Geometry: final body of the model. Coordinates: model frame, mm. A direction names the side the tool comes from. Give positions to 0.01 mm unless a question says otherwise; leave off trailing zeros. Write each loop counter-clockwise with the first axis right and the second up, starting at its lowest first coordinate (ties: lowest second). Pieces come first, ordered by that corner, then holes. Notation, with made-up numbers: M 54,14.25 L 109,14.25 A16 ccw 109,40.25 Z; hole C 33.25,18 d7. An arc over 180 degrees is marked long. Use a Markdown table: item, result. Add a question column.
(1) Reachability of faces 1 (the flat face through (2.2, 0, 0.1)), 2 (the cylindrical face through (0, 7, 5)), 3 (the cylindrical face through (-1.9, 4.3, -5.9)) from +Z, -Z, +X, -X, +Y, -Y: full face, straight path, thin tool, end or side. Return the list, or none.
(2) Material intervals for L1, parallel to X at y = 5.7, z = 0; L2, parallel to Z at x = -14, y = 24.5; L3, parallel to X at y = 19, z = -2.5, sorted ascending.
(3) Pin query (flat end, axial travel): pin 1 Ø16 at (x, z) = (0, 0) entering from +Y; pin 2 Ø12 at (x, y) = (-10.5, 13) entering from -Z; pin 3 Ø10 at (x, y) = (18, 26.5) entering from -Z. Return the tip coordinate at first contact, or that it passes through.
(4) Cut plane A-A (y = 19.25). Output: boundary loops of the cut face in (x, z).
(5) Cut plane B-B (y = 25). Output: boundary loops of the cut face in (x, z).
```python
from build123d import *

# Parameters (mm, degrees)
FILLET1_R = 5
FILLET2_R = 0.4
FILLET3_R = 1


with BuildPart() as part:
    # Sketch1 → Revolve1 (revolve)
    with BuildSketch(Plane.XY, mode=Mode.PRIVATE) as revolve1_sk:
        Polygon((5, 5.196152423), (5, 10), (25, 30), (26.697056275, 30), (6.2, 9.502943725), (6.2, 4.874613392), (6.2, 0), (2, 0), align=None)
    revolve(revolve1_sk.sketch.rotate(Axis((0, 0, 0), (0, 1, 0)), 90), axis=Axis((0, 0, 0), (0, 1, 0)))

    # Fillet1
    fillet1_edges = [part.edges().sort_by_distance(p)[0] for p in [
        (0, 9.502943725, 6.2),
        (0, 10, 5),
    ]]
    fillet(fillet1_edges, radius=FILLET1_R)

    # Fillet2
    fillet2_edges = [part.edges().sort_by_distance(p)[0] for p in [
        (0, 30, 26.697056275),
        (0, 30, 25),
    ]]
    fillet(fillet2_edges, radius=FILLET2_R)

    # Fillet3
    fillet3_edges = [part.edges().sort_by_distance(p)[0] for p in [
        (0, 0, 6.2),
    ]]
    fillet(fillet3_edges, radius=FILLET3_R)


solid = part.part
```
Answer list:
| question | item | result |
|---|---|---|
| 1 | face 1 | +Z, -Z, +X, -X, -Y |
| 1 | face 2 | +Y |
| 1 | face 3 | -Y |
| 2 | L1 | -6.2 to -5, 5 to 6.2 |
| 2 | L2 | -15.92 to -13.57, 13.57 to 15.92 |
| 2 | L3 | -15.5 to -13.77, 13.77 to 15.5 |
| 3 | pin 1 | y = 13 |
| 3 | pin 2 | z = -12.88 |
| 3 | pin 3 | z = -22.05 |
| 4 | outline | C 0,0 d31.89; hole C 0,0 d28.5 |
| 5 | outline | C 0,0 d43.39; hole C 0,0 d40 |
